CAD build for the part. Positions are in the model's coordinates, mm. Round coordinates to 2 decimals unless told otherwise and drop trailing zeros. Write each loop counter-clockwise with the first axis right and the second up, starting at its lowest first coordinate (ties: lowest second). Pieces come first, ordered by that corner, then holes. Notation, with made-up numbers: (11, 49.5) - (51, 49.5) arc R21 cw to (51, 69.5) - close; hole circle Ø1 at (-24.75, 68.25). An arc over 180 degrees is marked (long way). Answer in a Markdown table with one row per item.
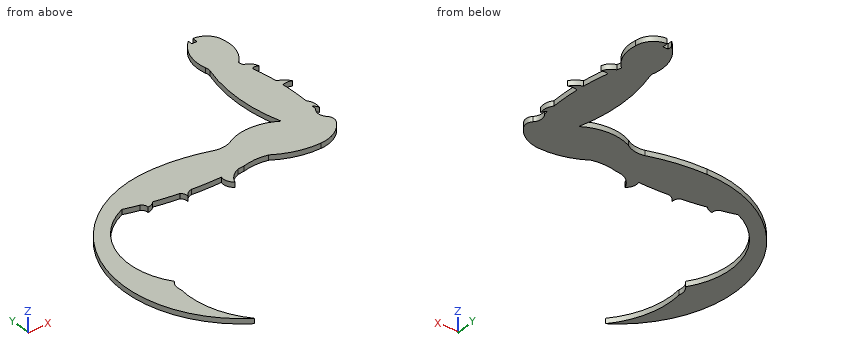
```python
from build123d import *

# Parameters (mm, degrees)
BOSS_EXTRUDE1_DEPTH = 1.524


with BuildPart() as part:
    # Sketch1 → Boss-Extrude1 (new body)
    with BuildSketch(Plane.XY):
        with BuildLine():
            Line((-1.524, 93.996264428), (0, 93.996264428))
            Line((0, 93.996264428), (0, 95.614927588))
            ThreePointArc((0, 95.614927588), (3.693748092, 94.060684173), (5.394313408, 90.431975702))
            ThreePointArc((5.394313408, 90.431975702), (5.083870366, 85.328096728), (2.344513216, 81.010472628))
            ThreePointArc((2.344513216, 81.010472628), (2.539372179, 80.361029228), (2.727630661, 79.709641871))
            ThreePointArc((2.727630661, 79.709641871), (4.432053028, 78.713510624), (5.394313408, 76.989739169))
            ThreePointArc((5.394313408, 76.989739169), (4.415817963, 77.356115064), (3.437322519, 76.989739169))
            ThreePointArc((3.437322519, 76.989739169), (4.210597619, 73.287177771), (4.773115775, 69.546791613))
            ThreePointArc((4.773115775, 69.546791613), (6.476278237, 68.669820648), (7.786173006, 67.271959374))
            ThreePointArc((7.786173006, 67.271959374), (6.398187856, 67.566469165), (5.010202706, 67.271959374))
            ThreePointArc((5.010202706, 67.271959374), (5.244344787, 62.991455343), (5.203509677, 58.704746843))
            ThreePointArc((5.203509677, 58.704746843), (6.122995482, 56.742128292), (6.022449708, 54.577130307))
            ThreePointArc((6.022449708, 54.577130307), (5.656055769, 55.32299802), (5.02447468, 55.863061433))
            ThreePointArc((5.02447468, 55.863061433), (4.967033142, 55.219803245), (4.903376867, 54.577130307))
            ThreePointArc((4.903376867, 54.577130307), (4.160208316, 52.476052404), (5.072854771, 50.442851897))
            ThreePointArc((5.072854771, 50.442851897), (5.82334848, 48.971843275), (5.510783631, 47.350297597))
            ThreePointArc((5.510783631, 47.350297597), (1.996073925, 43.775155466), (-2.817678827, 42.374223627))
            ThreePointArc((-2.817678827, 42.374223627), (-9.49417325, 43.186036631), (-15.638900273, 45.92043747))
            ThreePointArc((-15.638900273, 45.92043747), (-19.39296862, 46.30049438), (-23.12808354, 45.765341186))
            ThreePointArc((-23.12808354, 45.765341186), (-24.022277431, 45.671562771), (-24.917397051, 45.587076243))
            ThreePointArc((-24.917397051, 45.587076243), (-27.334149164, 44.07870078), (-28.883355756, 41.687917174))
            ThreePointArc((-28.883355756, 41.687917174), (-30.089948499, 43.281908325), (-30.179098122, 45.279087881))
            ThreePointArc((-30.179098122, 45.279087881), (-34.542573171, 45.266801777), (-38.901124358, 45.474399945))
            ThreePointArc((-38.901124358, 45.474399945), (-40.315710263, 44.818959656), (-41.31100161, 43.61893866))
            ThreePointArc((-41.31100161, 43.61893866), (-41.365656867, 44.810730455), (-42.081209312, 45.765371529))
            ThreePointArc((-42.081209312, 45.765371529), (-45.704386877, 46.241994184), (-49.304220896, 46.871104556))
            ThreePointArc((-49.304220896, 46.871104556), (-50.306617349, 46.062069726), (-51.560134873, 45.765371529))
            ThreePointArc((-51.560134873, 45.765371529), (-51.69154215, 46.839952524), (-52.498251339, 47.561902989))
            ThreePointArc((-52.498251339, 47.561902989), (-54.753856575, 48.126581404), (-56.993482586, 48.751635021))
            ThreePointArc((-56.993482586, 48.751635021), (-68.899192265, 35.07600442), (-65.606179776, 17.245556751))
            ThreePointArc((-65.606179776, 17.245556751), (-66.511011599, 15.524715569), (-66.48442613, 13.580671275))
            ThreePointArc((-66.48442613, 13.580671275), (-65.472964, 2.7909779), (-60.077247453, -6.607255003))
            ThreePointArc((-60.077247453, -6.607255003), (-74.778475075, 32.819889944), (-40.89052168, 57.764477873))
            ThreePointArc((-40.89052168, 57.764477873), (-32.596685646, 57.102075632), (-24.506779764, 55.157875102))
            ThreePointArc((-24.506779764, 55.157875102), (-21.512905256, 55.048508832), (-18.750408328, 56.207756982))
            ThreePointArc((-18.750408328, 56.207756982), (-11.598379652, 57.610020261), (-4.659613728, 55.380360214))
            ThreePointArc((-4.659613728, 55.380360214), (-6.824036174, 68.85301684), (-5.055416365, 82.38332301))
            ThreePointArc((-5.055416365, 82.38332301), (-4.963334277, 83.197390982), (-5.135176923, 83.998425237))
            ThreePointArc((-5.135176923, 83.998425237), (-4.912918532, 90.191927066), (-1.524, 95.380770374))
            Line((-1.524, 95.380770374), (-1.524, 93.996264428))
        make_face()
    extrude(amount=BOSS_EXTRUDE1_DEPTH)


solid = part.part
```
Q1. Flat gauge pins, fed straight in: pin 1 (0.5 mm diameter, centred on y = 94.5, z = 0.5, fed in from -X); pin 2 (0.8 mm diameter, centred on x = -0.5, z = 1, fed in from +Y); pin 3 (3 mm diameter, centred on x = -41.5, y = 60, fed in from +Z). Where does each tip first touch, or does it go through?
Computed:
| item | result |
|---|---|
| pin 1 | stops at x = -2.64 |
| pin 2 | stops at y = 94 |
| pin 3 | passes through |
Q2. Drill centre lines: line 1 (Y direction, x = -60.5, z = 1); line 2 (X direction, y = 80, z = 1.05); line 3 (Y direction, x = -25.5, z = 0.1). Where is each one in solid material? Low to high.
Computed:
| item | result |
|---|---|
| line 1 | y = -6.33 to -6.13, 46.83 to 52.02 |
| line 2 | x = -5.66 to 2.64 |
| line 3 | y = 45.35 to 55.47 |
Q3. Saw through at C-C on x = -45.5. List the corners of the cut face in (y, z).
Computed:
| item | result |
|---|---|
| outline | (46.21, 0) - (57.51, 0) - (57.51, 1.52) - (46.21, 1.52) - close |
Q4. Saw through at B-B on y = 34.5. List the corners of the cut face in (x, z), then the cut area to 3 significant figures.
Computed:
| item | result |
|---|---|
| outline | (-74.23, 0) - (-69.05, 0) - (-69.05, 1.52) - (-74.23, 1.52) - close |
| area | 7.90 mm2 |
Q5. Saw through at A-A on x = -63.5. List the corners of the cut face in (y, z).
Computed:
| item | result |
|---|---|
| outline | (-4.12, 0) - (-1.81, 0) - (-1.81, 1.52) - (-4.12, 1.52) - close; (44.35, 0) - (49.81, 0) - (49.81, 1.52) - (44.35, 1.52) - close |
